Read the model definition and answer for the solid it produces. Units are mm, in the model's axes. A direction names the side the tool comes from. Coordinates: 2 decimals unless noted, no trailing zeros. Loops run counter-clockwise (first coordinate to the right, second up) from the corner with the lowest first, then second, coordinate; pieces in that order, holes last. Notation, with made-up numbers: (42.25, 1) -> (75.25, 1) arc R26 cw to (75.25, 17) -> close; hole circle Ø6 at (44, 45). An arc over 180 degrees is marked (long way). Answer as a JSON object with one key per item and string values. Group by question number.
1) Flat-ended cylindrical pins translate along their axes: P1, Ø1.5, axis at x = 0.5, z = 0, coming from the -Y side; P2, Ø1, axis at y = 2.5, z = -2.5, coming from the -X side; P3, Ø1.5, axis at x = -0.5, y = 1, coming from the +Z side (3 decimals). Find the tip coordinate at first contact, or state that the pin passes through.
2) Section A-A, the plane z = 0 is taken. Give the vertices of the cut face in (x, y) (3 decimals).
3) Determine the mould class of faces 3 (the face through (-3, 0, -4)), 4 (the face through (0, 2.55, 0)), 5 (the face through (1.78, 1.31, 5.65)) for opening direction X: released by +X, released by -X, zero draft, split by the parting line, or undercut.
4) Section C-C, the plane y = 0.5 is taken. Give the vertices of the cut face in (x, z) (3 decimals).
5) Section B-B, the plane x = 0 is taken. Give the vertices of the cut face in (y, z) (3 decimals), plus the area to 3 significant figures.
6) Which of the six approach directions +Z, -Z, +X, -X, +Y, -Y give full straight-line access (tool end or side, diameter ignored) to faces 1 (the face through (-1.771, 1.257, 4.272)), 2 (the face through (0, 2.95, 0))?
7) Consider probe 1 along X at (y, z) = (0.95, 0) (3 decimals); probe 2 along X at (y, z) = (2, 3.5); probe 3 along Y at (x, z) = (-2.25, 3.25). Determine where each line is inside the solid, lowest interval first. Write a range as [from, to].
from build123d import *

# Parameters (mm, degrees)
SKETCH1_R           = 5.925
SKETCH1_R_2         = 4.625
BOSS_EXTRUDE1_DEPTH = 2.95
BOSS_EXTRUDE2_START = -0.4
SKETCH2_R           = 5.925
BOSS_EXTRUDE2_DEPTH = 0.4
FILLET1_R           = 0.3


with BuildPart() as part:
    # Sketch1 → Boss-Extrude1 (new body)
    with BuildSketch(Plane(origin=(0, 0, 0), x_dir=(1, 0, 0), z_dir=(0, 1, 0))):
        with Locations(Location((0, 0, 0), (0, 0, 270))):
            Circle(SKETCH1_R)
        with Locations(Location((0, 0, 0), (0, 0, 270))):
            Circle(SKETCH1_R_2, mode=Mode.SUBTRACT)
    extrude(amount=BOSS_EXTRUDE1_DEPTH)

    # Sketch2 → Boss-Extrude2 (add)
    with BuildSketch(Plane(origin=(0, 2.95, 0), x_dir=(1, 0, 0), z_dir=(0, 1, 0)).offset(BOSS_EXTRUDE2_START)):
        with Locations(Location((0, 0, 0), (0, 0, 270))):
            Circle(SKETCH2_R)
    extrude(amount=BOSS_EXTRUDE2_DEPTH)

    # Fillet1
    fillet1_edges = [part.edges().sort_by_distance(p)[0] for p in [
        (0, 2.95, -5.925),
    ]]
    fillet(fillet1_edges, radius=FILLET1_R)


solid = part.part
Determined:
{
 "1": {"P1": "y = 2.55", "P2": "x = -5.58", "P3": "z = 5.925"},
 "2": {"outline": "(-5.925, 0) -> (-4.625, 0) -> (-4.625, 2.55) -> (4.625, 2.55) -> (4.625, 0) -> (5.925, 0) -> (5.925, 2.65) arc R0.3 ccw to (5.625, 2.95) -> (-5.625, 2.95) arc R0.3 ccw to (-5.925, 2.65) -> close"},
 "3": {"face 3": "zero draft", "face 4": "undercut", "face 5": "split by the parting line"},
 "4": {"outline": "circle Ø11.85 at (0, 0); hole circle Ø9.25 at (0, 0)"},
 "5": {"outline": "(0, -5.925) -> (2.65, -5.925) arc R0.3 ccw to (2.95, -5.625) -> (2.95, 5.625) arc R0.3 ccw to (2.65, 5.925) -> (0, 5.925) -> (0, 4.625) -> (2.55, 4.625) -> (2.55, -4.625) -> (0, -4.625) -> close", "area": "11.3 mm²"},
 "6": {"face 1": "-Y", "face 2": "+Z, -Z, +X, -X, +Y"},
 "7": {"probe 1": "[-5.925, -4.625], [4.625, 5.925]", "probe 2": "[-4.78, -3.02], [3.02, 4.78]", "probe 3": "[2.55, 2.95]"}
}
